```python
from build123d import *

# Parameters (mm, degrees)
SKETCH_5_W               = 40
SKETCH_5_H               = 40
EXTRUDE_2_DEPTH          = 5
CUT_EXTRUDE_2_DEPTH      = 21
CUT_EXTRUDE_2_DEPTH_BACK = 21
SKETCH_7_R               = 1.7
CUT_EXTRUDE_4_DEPTH      = 6
CUT_EXTRUDE_4_DEPTH_BACK = 1
SKETCH_8_R               = 13.836233659
EXTRUDE_3_DEPTH          = 5
SKETCH_9_R               = 12.5
SKETCH_9_R_2             = 12
CUT_EXTRUDE_5_DEPTH      = 2.5
SKETCH_11_R              = 13
SKETCH_11_R_2            = 11.5
CUT_EXTRUDE_6_DEPTH      = 1.25
SKETCH_13_W              = 40
SKETCH_13_H              = 5
EXTRUDE_5_DEPTH          = 30


with BuildPart() as part:
    # Эскиз5 → Бобышка-Вытянуть2 (new body)
    with BuildSketch(Plane(origin=(0, 0, 0), x_dir=(1, 0, 0), z_dir=(0, 1, 0))):
        Rectangle(SKETCH_5_W, SKETCH_5_H)
    extrude(amount=EXTRUDE_2_DEPTH)

    # Эскиз6 → Вырез-Вытянуть2 (cut, two sides)
    with BuildSketch(Plane.XY) as cut_extrude_2_sk:
        Polygon((8.127281001, 0), (11.855143598, 3.727862597), (15.583006195, 0), align=None)
        Polygon((-8.127281001, 0), (-11.855143598, 3.727862597), (-15.583006195, 0), align=None)
    extrude(amount=CUT_EXTRUDE_2_DEPTH, mode=Mode.SUBTRACT)
    extrude(cut_extrude_2_sk.sketch, amount=-CUT_EXTRUDE_2_DEPTH_BACK, mode=Mode.SUBTRACT)

    # Эскиз7 → Вырез-Вытянуть4 (cut, two sides)
    with BuildSketch(Plane(origin=(0, 0, 0), x_dir=(1, 0, 0), z_dir=(0, 1, 0))) as cut_extrude_4_sk:
        with Locations((-17.5, -17.5)):
            Circle(SKETCH_7_R)
        with Locations((-17.5, 17.5)):
            Circle(SKETCH_7_R)
        with Locations((17.5, 17.5)):
            Circle(SKETCH_7_R)
        with Locations((17.5, -17.5)):
            Circle(SKETCH_7_R)
    extrude(amount=CUT_EXTRUDE_4_DEPTH, mode=Mode.SUBTRACT)
    extrude(cut_extrude_4_sk.sketch, amount=-CUT_EXTRUDE_4_DEPTH_BACK, mode=Mode.SUBTRACT)

    # Эскиз8 → Бобышка-Вытянуть3 (add)
    with BuildSketch(Plane(origin=(0, 5, 0), x_dir=(1, 0, 0), z_dir=(0, 1, 0))):
        Circle(SKETCH_8_R)
    extrude(amount=EXTRUDE_3_DEPTH)

    # Эскиз9 → Вырез-Вытянуть5 (cut)
    with BuildSketch(Plane(origin=(0, 10, 0), x_dir=(1, 0, 0), z_dir=(0, 1, 0))):
        Circle(SKETCH_9_R)
        Circle(SKETCH_9_R_2, mode=Mode.SUBTRACT)
    extrude(amount=-CUT_EXTRUDE_5_DEPTH, mode=Mode.SUBTRACT)

    # Эскиз11 → Вырез-Вытянуть6 (cut)
    with BuildSketch(Plane(origin=(0, 7.5, 0), x_dir=(1, 0, 0), z_dir=(0, 1, 0))):
        Circle(SKETCH_11_R)
        Circle(SKETCH_11_R_2, mode=Mode.SUBTRACT)
    extrude(amount=CUT_EXTRUDE_6_DEPTH, mode=Mode.SUBTRACT)

    # Эскиз13 → Бобышка-Вытянуть5 (add)
    with BuildSketch(Plane(origin=(0, 0, 0), x_dir=(1, 0, 0), z_dir=(0, 1, 0))):
        with Locations((0, 22.5)):
            Rectangle(SKETCH_13_W, SKETCH_13_H)
    extrude(amount=EXTRUDE_5_DEPTH)


solid = part.part
```
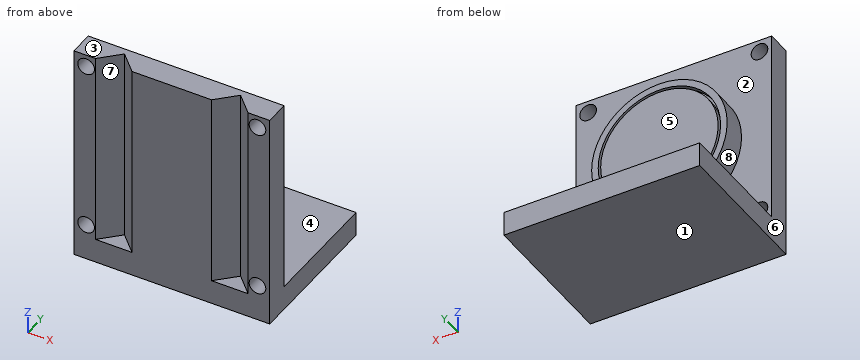
For this review, take the finished solid that the model builds, in its own axes (mm). Face numbers are marked on the shaded views. A direction names the side the tool comes from. Coordinates: 2 decimals unless noted, no trailing zeros. Order: outer loops, then holes, each group sorted by start corner. A loop starts at its lowest first (then second) coordinate and runs counter-clockwise, first axis right, second up. Notation, with made-up numbers: (11.25, 23) - (24.25, 23) arc R20 ccw to (24.25, 55) - close; hole circle Ø3 at (23, 20.5). An arc over 180 degrees is marked (long way). Answer as a JSON object with one key per item and string values. Group by question number.
1. We need section B-B on y = 5.75. State the section outline as (x, z) points, then the cut area to 3 significant figures.
2. Clearance check with flat-ended pins moving along their axes: P1, Ø12, axis at x = -1, z = -1.5, coming from the +Y side; P2, Ø4, axis at x = -17.5, z = -17.5, coming from the +Y side; P3, Ø3, axis at y = 7, z = -12, coming from the +X side; P4, Ø10, axis at y = 18.5, z = -8.5, coming from the -X side. State where each tip first meets the part, or that it passes through.
3. The part is to be moulded in two halves that separate along Z. For the marked faces 1, 2 and 3, say which applies: pulls with the +Z half, pulls with the -Z half, needs draft (parallel to the pull), parting line crosses it, or undercut.
4. For probe 1 along Z at (x, y) = (-17.5, 2.45); probe 2 along Z at (x, y) = (0, 9.2); probe 3 along X at (y, z) = (3.85, 17.5), list the stretches that pass through material, from the lowest coordinate up.
5. For the marked faces 4, 5, 6, 7 and 8, list the 3-axis set-ups (+Z, -Z, +X, -X, +Y, -Y) from which the entire face can be reached by the end or side of a thin tool; tool diameter is ignored.
6. We need section A-A on x = -17.5. State the section outline as (y, z) points.
7. We need section D-D on x = 0. State the section outline as (y, z) points.
Final values:
{
 "1": {"outline": "(-20, -25) - (20, -25) - (20, -20) - (-20, -20) - close; circle Ø27.67 at (0, 0)", "area": "801 mm²"},
 "2": {"P1": "y = 10", "P2": "y = 5", "P3": "x = 9.01", "P4": "through"},
 "3": {"face 1": "pulls with the -Z half", "face 2": "undercut", "face 3": "pulls with the +Z half"},
 "4": {"probe 1": "-25 to -19.2, -15.8 to 15.8, 19.2 to 20", "probe 2": "-25 to -20, -13.84 to -12.5, -12 to 12, 12.5 to 13.84", "probe 3": "-20 to -19.2, -15.8 to 15.8, 19.2 to 20"},
 "5": {"face 4": "+X, -X, +Y", "face 5": "+Z, +X, -X, +Y", "face 6": "+Z, -Z, -X, +Y, -Y", "face 7": "+Z, -Y", "face 8": "+Y"},
 "6": {"outline": "(0, -25) - (30, -25) - (30, -20) - (5, -20) - (5, -19.2) - (0, -19.2) - close; (0, -15.8) - (5, -15.8) - (5, 15.8) - (0, 15.8) - close; (0, 19.2) - (5, 19.2) - (5, 20) - (0, 20) - close"},
 "7": {"outline": "(0, -25) - (30, -25) - (30, -20) - (5, -20) - (5, -13.84) - (10, -13.84) - (10, -12.5) - (8.75, -12.5) - (8.75, -13) - (7.5, -13) - (7.5, -11.5) - (8.75, -11.5) - (8.75, -12) - (10, -12) - (10, 12) - (8.75, 12) - (8.75, 11.5) - (7.5, 11.5) - (7.5, 13) - (8.75, 13) - (8.75, 12.5) - (10, 12.5) - (10, 13.84) - (5, 13.84) - (5, 20) - (0, 20) - close"}
}
